CAD build for the part. Positions are in the model's coordinates, mm. A direction names the side the tool comes from. Coordinates: 2 decimals unless noted, no trailing zeros. Loops run counter-clockwise (first coordinate to the right, second up) from the corner with the lowest first, then second, coordinate; pieces in that order, holes last. Notation, with made-up numbers: (-36.75, -26.75) -> (22.25, -26.75) arc R31 cw to (22.25, -1.75) -> close; hole circle Ø10 at (38.5, 25.25). An arc over 180 degrees is marked (long way). Write each question's results on one line, items separated by ' | '.
```python
from build123d import *

# Parameters (mm, degrees)
F2_R     = 5.125
F3_DEPTH = 1.5
F4_R     = 2.35
F5_DEPTH = 3.5


with BuildPart() as f1:
    # F0 (on Front) → F1 (revolve)
    with BuildSketch(Plane.XZ):
        with BuildLine():
            ThreePointArc((0, 1.511369), (-3.807453, 1.861515), (-7.487184, 2.900208))
            ThreePointArc((-7.487184, 2.900208), (-9.5, 1.773576), (-8.025159, 0))
            Line((-8.025159, 0), (0, 0))
            Line((0, 0), (0, 1.511369))
        make_face()
    revolve(axis=Axis((0, 0, 0.755685), (0, 0, 1)))

    # F2 (on Top) → F3 (join)
    with BuildSketch(Plane.XY):
        Circle(F2_R)
    extrude(amount=-F3_DEPTH)

    # F4 (on Top) → F5 (join)
    with BuildSketch(Plane.XY):
        Circle(F4_R)
    extrude(amount=-F5_DEPTH)


solid = f1.part
```
Q1. Wall check: L1, parallel to Z at x = 5, y = 6.25; L2, parallel to Y at x = 0, z = -0.25 (3 decimals); L3, parallel to Y at x = -2, z = 1. Give the ranges that are in metal, low to high. Write a range as from..to.
Results are:
L1: 0..3 | L2: -5.125..5.125 | L3: -9.23..9.23
Q2. Which spindle directions (+Z, -Z, +X, -X, +Y, -Y) get a long thin tool onto all of the face, cutting with end or side? Do faces 1 (the flat face through (0, 0, -3.5)), 2 (the flat face through (2.2, 1.2, -1.5)). Say none if no direction does.
Results are:
face 1: -Z, +X, -X, +Y, -Y | face 2: -Z
Q3. Cut at B-B on z = 0.5. Write the cut outline in (x, y), and give its area (3 significant figures).
Results are:
outline: circle Ø18.29 at (0, 0) | area: 263 mm^2
Q4. Drop flat-ended pins along their axis: pin 1 (2 mm diameter, centred on x = -6, y = -0.5, fed in from -Z); pin 2 (2 mm diameter, centred on y = -2.5, z = -0.5, fed in from +X); pin 3 (2 mm diameter, centred on x = 3.5, z = 1.5, fed in from +Y). Give the stop position or say it passes through.
Results are:
pin 1: z = -1.5 | pin 2: x = 8.83 | pin 3: y = 9.19
Q5. Cut at A-A on z = -2.5. Write the cut outline in (x, y), and give its area (3 significant figures).
Results are:
outline: circle Ø4.7 at (0, 0) | area: 17.3 mm^2
